```python
from build123d import *

# Parameters (mm, degrees)
SKETCH1_R             = 92.5
BOSS_EXTRUDE1_DEPTH   = 10
SKETCH2_R             = 15
CUT_EXTRUDE1_DEPTH    = 132.196417634
SKETCH3_R             = 6.837022299
CUT_EXTRUDE2_DEPTH    = 8.466961
CIRPATTERN1_START     = 1.53303864
CIRPATTERN1_OUTLINE_R = 6.837022299
CIRPATTERN1_DEPTH     = 8.46696136


# Read off the part's stored shape, not the designer's step: CirPattern1
with BuildPart() as part:
    # Sketch1 → Boss-Extrude1 (new body)
    with BuildSketch(Plane(origin=(0, 0, 0), x_dir=(1, 0, 0), z_dir=(0, 1, 0))):
        with Locations(Location((0, 0, 0), (0, 0, 270))):
            Circle(SKETCH1_R)
    extrude(amount=BOSS_EXTRUDE1_DEPTH)

    # Sketch2 → Cut-Extrude1 (cut, through all)
    with BuildSketch(Plane(origin=(0, 0, 0), x_dir=(1, 0, 0), z_dir=(0, 1, 0))):
        with Locations(Location((0, 0, 0), (0, 0, 270))):
            Circle(SKETCH2_R)
    extrude(amount=CUT_EXTRUDE1_DEPTH, mode=Mode.SUBTRACT)

    # Sketch3 → Cut-Extrude2 (cut)
    with BuildSketch(Plane(origin=(0, 10, 0), x_dir=(1, 0, 0), z_dir=(0, 1, 0))):
        with Locations(Location((-27.649021732, 0, 0), (0, 0, 270))):
            Circle(SKETCH3_R)
    extrude(amount=-CUT_EXTRUDE2_DEPTH, mode=Mode.SUBTRACT)

    # CirPattern1 outline → CirPattern1 (cut)
    with BuildSketch(Plane(origin=(0, 0, 0), x_dir=(1, 0, 0), z_dir=(0, 1, 0)).offset(CIRPATTERN1_START)):
        with Locations((-19.55081076, -19.55081076)):
            Circle(CIRPATTERN1_OUTLINE_R)
        with Locations((-19.55081076, 19.55081076)):
            Circle(CIRPATTERN1_OUTLINE_R)
        with Locations((0, 27.649021732)):
            Circle(CIRPATTERN1_OUTLINE_R)
        with Locations((19.55081076, 19.55081076)):
            Circle(CIRPATTERN1_OUTLINE_R)
        with Locations((27.649021732, 0)):
            Circle(CIRPATTERN1_OUTLINE_R)
        with Locations((19.55081076, -19.55081076)):
            Circle(CIRPATTERN1_OUTLINE_R)
        with Locations((0, -27.649021732)):
            Circle(CIRPATTERN1_OUTLINE_R)
    extrude(amount=CIRPATTERN1_DEPTH, mode=Mode.SUBTRACT)


solid = part.part
```
Geometry check sheet. Reference: the model listing, model coordinates, mm. A direction names the side the tool comes from. Coordinates: 2 decimals unless noted, no trailing zeros. Loops run counter-clockwise (first coordinate to the right, second up) from the corner with the lowest first, then second, coordinate; pieces in that order, holes last. Notation, with made-up numbers: (-26.5, 5.5) - (30.5, 5.5) arc R20 cw to (30.5, 37.5) - close; hole circle Ø6 at (6, -24). An arc over 180 degrees is marked (long way). One line per item, written item: value. Start each with the question number.
(1) Mould release check, pull along Z, two halves, no side actions. Record for faces 1 (the flat face through (19, 1.533, -20)), 2 (the cylindrical face through (-20.44, 5.71, 12.77)), 3 (the flat face through (-19, 10, -1)), 4 (the cylindrical face through (-90.3, 4.93, -20.05)): released by +Z, released by -Z, zero draft, split by the parting line, or undercut.
(2) Cross-section at D-D on x = 50. Enter the section's corners in (y, z).
(3) Cross-section at C-C on y = 5.75. Count the separate pieces of the cut face and the enclosed holes in it, plus the area to 3 significant figures.
(4) Depth check by flat-ended pin: P1, Ø5, axis at y = 8, z = 70, coming from the -X side; P2, Ø24, axis at x = 0, z = 0, coming from the +Y side; P3, Ø3, axis at x = 54.5, y = 4.5, coming from the -Z side; P4, Ø4, axis at x = -26.5, z = 1.5, coming from the +Y side. Enter the tip coordinate at first touch or a pass-through.
(5) Tool access check on faces 5 (the cylindrical face through (33.965, 5.707, 2.619)), 6 (the flat face through (-19, 0, -1)). Record the directions out of +Z, -Z, +X, -X, +Y, -Y that give a thin tool (end or side, any length) a straight path to the whole face; none if there is none.
(6) Cross-section at A-A on x = 0. Enter the section's corners in (y, z).
(7) Cross-section at B-B on z = 0. Enter the section's corners in (x, y).
(8) Material ranges on line 1 (X direction, y = 8.25, z = 0); line 2 (Z direction, x = -17, y = 5.75); line 3 (Z direction, x = 18, y = 9.25), recorded low to high. Write a range as [from, to].
Results below:
1. face 1: undercut
1. face 2: undercut
1. face 3: zero draft
1. face 4: split by the parting line
2. outline: (0, -77.82) - (10, -77.82) - (10, 77.82) - (0, 77.82) - close
3. separate pieces: 1
3. enclosed holes: 9
3. area: 25,000 mm2
4. P1: stops at x = -63.25
4. P2: passes through
4. P3: stops at z = -75.81
4. P4: stops at y = 1.53
5. face 5: +Y
5. face 6: +Z, -Z, +X, -X, -Y
6. outline: (0, -92.5) - (10, -92.5) - (10, -34.49) - (1.53, -34.49) - (1.53, -20.81) - (10, -20.81) - (10, -15) - (0, -15) - close; (0, 15) - (10, 15) - (10, 20.81) - (1.53, 20.81) - (1.53, 34.49) - (10, 34.49) - (10, 92.5) - (0, 92.5) - close
7. outline: (-92.5, 0) - (-15, 0) - (-15, 10) - (-20.81, 10) - (-20.81, 1.53) - (-34.49, 1.53) - (-34.49, 10) - (-92.5, 10) - close; (15, 0) - (92.5, 0) - (92.5, 10) - (34.49, 10) - (34.49, 1.53) - (20.81, 1.53) - (20.81, 10) - (15, 10) - close
8. line 1: x = [-92.5, -34.49], [-20.81, -15], [15, 20.81], [34.49, 92.5]
8. line 2: z = [-90.92, -25.89], [-13.21, 13.21], [25.89, 90.92]
8. line 3: z = [-90.73, -26.21], [-12.89, 12.89], [26.21, 90.73]
